Autodesk Inventor part; units mm, degrees
ref_plane "YZ Plane" through (0, 0, 0) normal (1, 0, 0) x (0, 1, 0)
ref_plane "XZ Plane" through (0, 0, 0) normal (0, 1, 0) x (-1, 0, 0)
ref_plane "XY Plane" through (0, 0, 0) normal (0, 0, 1) x (1, 0, 0)
sketch "Sketch1" plane through (0, 0, 0) normal (0, 0, 1) x (1, 0, 0)
  line L0 (25, 0) -> (35, 0)
  line L1 (35, 0) -> (35, 5)
  line L2 (25, 0) -> (25, 5)
  arc A0 (27, 5) -> (33, 5) centre (30, 5) ccw
  line L3 (35, 5) -> (33, 5)
  line L4 (25, 5) -> (27, 5)
  line L5 (0, -1) -> (0, 6)
  point P0 (0, 0)
  point P1 (30, 0)
  dimension "d0" = 25
  dimension "d1" = 10
  dimension "d2" = 5
  dimension "d3" = 6
revolve "Revolution1" add sketch "Sketch1" angle 360 about axis through (0, -10, 0) along (0, 1, 0)
chamfer "Chamfer1" distance 0.2 angle 45 6 edges at (-25, 0, 0) (-35, 0, 0) (-35, 5, 0) (-33, 5, 0) (-27, 5, 0) (-25, 5, 0)
properties part number "UBC Bearing 51110 - buitenkant" material "Stainless Steel"
Build history of the part. All positions in model axes, mm. Give positions to 0.01 mm unless a question says otherwise; leave off trailing zeros. Order: outer loops, then holes, each group sorted by start corner. A loop starts at its lowest first (then second) coordinate and runs counter-clockwise, first axis right, second up. Notation, with made-up numbers: M -5.75,40.5 L 33.25,40.5 A9 cw 33.25,44.5 Z; hole C 47.5,60 d8. An arc over 180 degrees is marked long. Return JSON: item names as keys, results as strings.
Q1. Wall check: probe 1 along X at (y, z) = (2.45, 18.5); probe 2 along X at (y, z) = (3.75, 0); probe 3 along Z at (x, y) = (0, 1.85). Give the ranges that are in metal, low to high. Write a range as from..to.
Answer list:
{"probe 1": "x = -29.71..-25.59, -21.57..-16.82, 16.82..21.57, 25.59..29.71", "probe 2": "x = -35..-32.73, -27.27..-25, 25..27.27, 32.73..35", "probe 3": "z = -35..-25, 25..35"}
Q2. Two-plate mould, pull along X, no slides. Class faces 1 (the face through (23.846, 2.532, -7.509)), 2 (the face through (-2.74, 5, -33.25)), 3 (the face through (-28, 3, 21)): pulls with the +X half, pulls with the -X half, needs draft (parallel to the pull), parting line crosses it, or undercut.
Answer list:
{"face 1": "undercut", "face 2": "needs draft", "face 3": "parting line crosses it"}
Q3. Band-saw the part on A-A (y = 3.45). Give the cut face in (x, z), then the cut area to 3 significant figures.
Answer list:
{"outline": "C 0,0 d70; C 0,0 d54.86; hole C 0,0 d65.14; hole C 0,0 d50", "area": "917 mm^2"}
Q4. Flat gauge pins, fed straight in: pin 1 (1.5 mm diameter, centred on y = 3, z = -3.5, fed in from -X); pin 2 (1 mm diameter, centred on x = -1.5, y = 2.5, fed in from +Z); pin 3 (10 mm diameter, centred on x = -11, z = -16, fed in from -Y); pin 4 (1.5 mm diameter, centred on x = -17, y = 1, fed in from +Z). Where does each tip first touch, or does it go through?
Answer list:
{"pin 1": "stops at x = -34.89", "pin 2": "stops at z = 34.99", "pin 3": "passes through", "pin 4": "stops at z = 31"}
